Source: CAD feature listing. Evaluate the final solid. Frame: model axes, mm. A direction names the side the tool comes from. Coordinates: 2 decimals unless noted, no trailing zeros. Order: outer loops, then holes, each group sorted by start corner. A loop starts at its lowest first (then second) coordinate and runs counter-clockwise, first axis right, second up.
```python
from build123d import *

# Parameters (mm, degrees)
MAIN_DEPTH            = 2.5
ESQUISSE2_R           = 2.5
ORIGINALBRACKET_DEPTH = 2
ESQUISSE3_R           = 1.3
FIXINGHOLE_DEPTH      = 5.5
LPATTERN1_COUNT       = 6
LPATTERN1_PITCH       = 5


with BuildPart() as part:
    # Esquisse1 → Main (new body)
    with BuildSketch(Plane.XY):
        with BuildLine():
            Line((-4.375785644, 4.25), (-6.426543071, 6.300757427))
            ThreePointArc((-6.426543071, 6.300757427), (-3.150224217, 8.43066352), (0.72, 8.971153772))
            Line((0.72, 8.971153772), (50.4, 4.983974318))
            ThreePointArc((50.4, 4.983974318), (55, 0), (50.4, -4.983974318))
            Line((50.4, -4.983974318), (0.72, -8.971153772))
            ThreePointArc((0.72, -8.971153772), (-3.150224217, -8.43066352), (-6.426543071, -6.300757427))
            Line((-6.426543071, -6.300757427), (-4.375785644, -4.25))
            ThreePointArc((-4.375785644, -4.25), (0, -6.1), (4.375785644, -4.25))
            Line((4.375785644, -4.25), (17.31559729, -2.78215714))
            ThreePointArc((17.31559729, -2.78215714), (19.8, 0), (17.31559729, 2.78215714))
            Line((17.31559729, 2.78215714), (4.375785644, 4.25))
            ThreePointArc((4.375785644, 4.25), (0, 6.1), (-4.375785644, 4.25))
        make_face()
    extrude(amount=MAIN_DEPTH)

    # Esquisse2 → OriginalBracket (add)
    with BuildSketch(Plane(origin=(0, 0, 0), x_dir=(-1, 0, 0), z_dir=(0, 0, -1))):
        with BuildLine():
            Line((-0.72, -8.971153772), (-50.4, -4.983974318))
            ThreePointArc((-50.4, -4.983974318), (-55, 0), (-50.4, 4.983974318))
            Line((-50.4, 4.983974318), (-0.72, 8.971153772))
            ThreePointArc((-0.72, 8.971153772), (3.150224217, 8.43066352), (6.426543071, 6.300757427))
            Line((6.426543071, 6.300757427), (6.426543071, -6.300757427))
            ThreePointArc((6.426543071, -6.300757427), (3.150224217, -8.43066352), (-0.72, -8.971153772))
        make_face()
        Circle(ESQUISSE2_R, mode=Mode.SUBTRACT)
    extrude(amount=ORIGINALBRACKET_DEPTH)

    # Esquisse3 → FixingHole (cut, through all)
    with BuildSketch(Plane.XY.offset(2.5)):
        with Locations((50, 0)):
            Circle(ESQUISSE3_R)
    fixinghole = extrude(amount=-FIXINGHOLE_DEPTH, mode=Mode.SUBTRACT)

    # LPattern1: FixingHole ×6
    with Locations(*[(-i * LPATTERN1_PITCH, 0, 0) for i in range(1, LPATTERN1_COUNT)]):
        add(fixinghole, mode=Mode.SUBTRACT)


solid = part.part
```
1. Section query C-C, the plane z = 1.3. Output: boundary loops of the cut face in (x, y), plus the area to 3 significant figures.
2. Draft query along X for faces 4 (the flat face through (17, 0, -2)), 5 (the flat face through (-5.387, 5.261, 1.232)), 6 (the cylindrical face through (0.1, 6.1, 1.2)). Return one class per face: +X half, -X half, draft (parallel to the pull), parting line (faces both ways), or undercut.
3. Section query B-B, the plane y = 0.75. Count the separate pieces of the cut face and the enclosed holes in it, plus the area to 3 significant figures.
4. Section query A-A, the plane x = 0. Output: boundary loops of the cut face in (y, z), plus the area to 3 significant figures.
5. Contact query for flat-ended pins moving along their axis: P1, Ø1, axis at x = 18, z = -1, coming from the -Y side; P2, Ø4, axis at x = 30, y = 0, coming from the -Z side; P3, Ø2, axis at x = 6, y = -1.5, coming from the +Z side. Output: stop coordinate, or through.
6. Material intervals for line 1 along Y through (x, z) = (0, -1.15); line 2 along Z through (x, y) = (6.5, -1.5); line 3 along Y through (x, z) = (7.5, 0.6), sorted ascending.
7. Access query for faces 1 (the cylindrical face through (33.7, 0.06, 0.28)), 2 (the cylindrical face through (-0.1, -6.1, 1.2)), 3 (the flat face through (10.936, 3.506, 1.232)). Directions: +Z, -Z, +X, -X, +Y, -Y. A direction counts if a zero-diameter tool reaches every point of the face in a straight line with its end or side. Return the directions, or none.
8. Section query D-D, the plane x = 39.5. Output: boundary loops of the cut face in (y, z), plus the area to 3 significant figures.
Answer key:
1. outline: (-6.43, -6.3) arc R9 ccw to (0.72, -8.97) - (50.4, -4.98) arc R5 ccw to (50.4, 4.98) - (0.72, 8.97) arc R9 ccw to (-6.43, 6.3) - (-4.38, 4.25) arc R6.1 cw to (4.38, 4.25) - (17.32, 2.78) arc R2.8 cw to (17.32, -2.78) - (4.38, -4.25) arc R6.1 cw to (-4.38, -4.25) - close; hole circle Ø2.6 at (25, 0); hole circle Ø2.6 at (30, 0); hole circle Ø2.6 at (35, 0); hole circle Ø2.6 at (40, 0); hole circle Ø2.6 at (45, 0); hole circle Ø2.6 at (50, 0)
1. area: 595 mm2
2. face 4: draft
2. face 5: -X half
2. face 6: undercut
3. separate pieces: 8
3. enclosed holes: 0
3. area: 144 mm2
4. outline: (-9, -2) - (-2.5, -2) - (-2.5, 0) - (-6.1, 0) - (-6.1, 2.5) - (-9, 2.5) - close; (2.5, -2) - (9, -2) - (9, 2.5) - (6.1, 2.5) - (6.1, 0) - (2.5, 0) - close
4. area: 40.5 mm2
5. P1: stops at y = -7.62
5. P2: stops at z = -2
5. P3: stops at z = 0
6. line 1: y = -9 to -2.5, 2.5 to 9
6. line 2: z = -2 to 0
6. line 3: y = -8.43 to -3.9, 3.9 to 8.43
7. face 1: +Z, -Z
7. face 2: +Z
7. face 3: +Z, -X
8. outline: (-5.86, -2) - (-1.2, -2) - (-1.2, 2.5) - (-5.86, 2.5) - close; (1.2, -2) - (5.86, -2) - (5.86, 2.5) - (1.2, 2.5) - close
8. area: 41.9 mm2
